```python
from build123d import *

# Parameters (mm, degrees)
SKETCH1_W           = 60
SKETCH1_H           = 60
BOSS_EXTRUDE1_DEPTH = 5
SKETCH2_R           = 2
CUT_EXTRUDE1_DEPTH  = 43.720018727
SKETCH5_R           = 2
CUT_EXTRUDE2_DEPTH  = 43.720018727
SKETCH6_R           = 2
CUT_EXTRUDE3_DEPTH  = 43.720018727
SKETCH7_R           = 2
CUT_EXTRUDE4_DEPTH  = 43.720018727
SKETCH8_W           = 5.522489043
SKETCH8_H           = 35.05943801
BOSS_EXTRUDE2_DEPTH = 4
SKETCH11_W          = 5.020444584
SKETCH11_H          = 34.724741706
BOSS_EXTRUDE3_DEPTH = 4


with BuildPart() as part:
    # Sketch1 → Boss-Extrude1 (new body)
    with BuildSketch(Plane.XY):
        Rectangle(SKETCH1_W, SKETCH1_H)
    extrude(amount=-BOSS_EXTRUDE1_DEPTH)

    # Sketch2 → Cut-Extrude1 (cut, through all)
    with BuildSketch(Plane.XY):
        with Locations((-26.441008142, 26.817541486)):
            Circle(SKETCH2_R)
    extrude(amount=-CUT_EXTRUDE1_DEPTH, mode=Mode.SUBTRACT)

    # Sketch5 → Cut-Extrude2 (cut, through all)
    with BuildSketch(Plane.XY):
        with Locations((-26.441008142, -26.231822951)):
            Circle(SKETCH5_R)
    extrude(amount=-CUT_EXTRUDE2_DEPTH, mode=Mode.SUBTRACT)

    # Sketch6 → Cut-Extrude3 (cut, through all)
    with BuildSketch(Plane.XY):
        with Locations((25.855289607, 26.817541486)):
            Circle(SKETCH6_R)
    extrude(amount=-CUT_EXTRUDE3_DEPTH, mode=Mode.SUBTRACT)

    # Sketch7 → Cut-Extrude4 (cut, through all)
    with BuildSketch(Plane.XY):
        with Locations((25.855289607, -26.231822951)):
            Circle(SKETCH7_R)
    extrude(amount=-CUT_EXTRUDE4_DEPTH, mode=Mode.SUBTRACT)

    # Sketch8 → Boss-Extrude2 (add)
    with BuildSketch(Plane.XY):
        with Locations((-13.555200377, 0)):
            Rectangle(SKETCH8_W, SKETCH8_H)
    extrude(amount=BOSS_EXTRUDE2_DEPTH)

    # Sketch11 → Boss-Extrude3 (add)
    with BuildSketch(Plane.XY):
        with Locations((13.4715263, 0)):
            Rectangle(SKETCH11_W, SKETCH11_H)
    extrude(amount=BOSS_EXTRUDE3_DEPTH)


solid = part.part
```
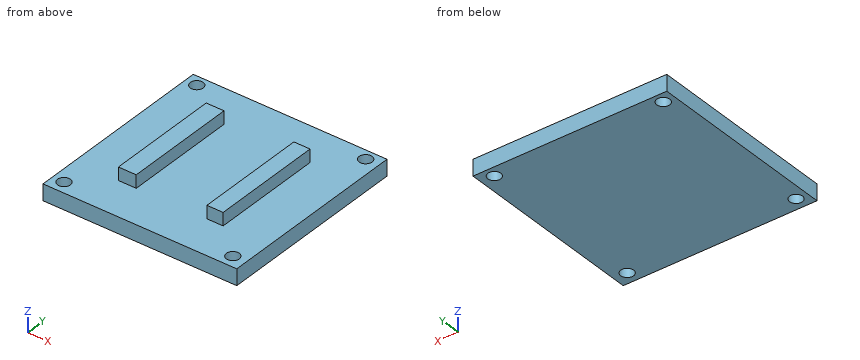
Work out the finished part from the listing and answer in its coordinate system (mm). Coordinates: 2 decimals unless noted, no trailing zeros. Write each loop counter-clockwise with the first axis right and the second up, starting at its lowest first coordinate (ties: lowest second). Pieces come first, ordered by that corner, then holes.
Q1. A cutting plane is placed at A-A, the plane z = 2.75. Give the vertices of the cut face in (x, y), then the cut area to 3 significant figures.
Q2. Each of these flat-tipped pins is pushed along its axis until it touches: pin 1 Ø2 at (y, z) = (-4, 2) entering from -X; pin 2 Ø5 at (x, y) = (3, -9) entering from +Z; pin 3 Ø4.5 at (y, z) = (1, 1.5) entering from +X; pin 4 Ø2 at (x, z) = (-13, 2) entering from -Y. Where does it stop, or does it pass through?
Q3. A cutting plane is placed at D-D, the plane x = -3. Give the vertices of the cut face in (y, z), then the cut area to 3 significant figures.
Q4. Find the intervals of material crossed by line 1 (X direction, y = -17, z = 1.25); line 2 (Z direction, x = 20, y = -6.5); line 3 (Y direction, x = -15, z = 3), in increasing order.
Q5. A cutting plane is placed at C-C, the plane y = 16. Give the vertices of the cut face in (x, z), then the cut area to 3 significant figures.
Q6. A cutting plane is placed at B-B, the plane x = -13. Give the vertices of the cut face in (y, z).
Findings below:
1. outline: (-16.32, -17.53) - (-10.79, -17.53) - (-10.79, 17.53) - (-16.32, 17.53) - close; (10.96, -17.36) - (15.98, -17.36) - (15.98, 17.36) - (10.96, 17.36) - close
1. area: 368 mm2
2. pin 1: stops at x = -16.32
2. pin 2: stops at z = 0
2. pin 3: stops at x = 30
2. pin 4: stops at y = -17.53
3. outline: (-30, -5) - (30, -5) - (30, 0) - (-30, 0) - close
3. area: 300 mm2
4. line 1: x = -16.32 to -10.79, 10.96 to 15.98
4. line 2: z = -5 to 0
4. line 3: y = -17.53 to 17.53
5. outline: (-30, -5) - (30, -5) - (30, 0) - (15.98, 0) - (15.98, 4) - (10.96, 4) - (10.96, 0) - (-10.79, 0) - (-10.79, 4) - (-16.32, 4) - (-16.32, 0) - (-30, 0) - close
5. area: 342 mm2
6. outline: (-30, -5) - (30, -5) - (30, 0) - (17.53, 0) - (17.53, 4) - (-17.53, 4) - (-17.53, 0) - (-30, 0) - close
